Model file for the job. Use its own axes, mm. Round coordinates to 2 decimals unless told otherwise and drop trailing zeros. Write each loop counter-clockwise with the first axis right and the second up, starting at its lowest first coordinate (ties: lowest second). Pieces come first, ordered by that corner, then holes. Notation, with made-up numbers: (-10, 43.5) - (31, 43.5) arc R21 cw to (31, 48.5) - close; hole circle Ø4 at (72, 80). An arc over 180 degrees is marked (long way). One line per item, written item: value.
Autodesk Inventor part; units mm, degrees
ref_plane "YZ Plane" through (0, 0, 0) normal (1, 0, 0) x (0, 1, 0)
ref_plane "XZ Plane" through (0, 0, 0) normal (0, 1, 0) x (-1, 0, 0)
ref_plane "XY Plane" through (0, 0, 0) normal (0, 0, 1) x (1, 0, 0)
sketch "Эскиз1" plane through (0, 0, 0) normal (0, 1, 0) x (-1, 0, 0)
  line L0 (0, 0) -> (30, 0)
  line L1 (30, 0) -> (30, -50)
  line L2 (30, -50) -> (0, -50)
  line L3 (0, -50) -> (0, 0)
  dimension "d0" = 30
  dimension "d1" = 50
extrude "Выдавливание1" add sketch "Эскиз1" along normal blind 15
fillet "Сопряжение1" radius 2 1 edges at (-15, 0, 0)
sketch "Эскиз2" plane through (0, 15, 0) normal (0, 1, 0) x (1, 0, 0)
  line L0 (-30, 0) -> (0, 0)
  point P0 (-15, 20)
  point P1 (-15, 0)
  dimension "d5" = 20
hole "Отверстие1" at (-15, 15, -20) direction (0, -1, 0) diameter 8 end through all
sketch "Эскиз3" plane through (0, 15, 0) normal (0, 1, 0) x (1, 0, 0)
  line L0 (-30, 0) -> (0, 0)
  circle A0 centre (-15, 20) radius 4
  line L1 (-30, 0) -> (0, 0)
  line L2 (0, 0) -> (0, 50)
  line L3 (0, 50) -> (-30, 50)
  line L4 (-30, 50) -> (-30, 0)
  line L5 (-30, 50) -> (-30, 0)
  line L6 (0, 0) -> (0, 50)
  point P0 (-30, 40)
  point P1 (0, 40)
  dimension "d13" = 40
hole "Отверстие2" at (-30, 15, -40) at (0, 15, -40) direction (0, -1, 0) diameter 2 end through all
sketch "Эскиз4" plane through (0, 2, 0) normal (1, 0, 0) x (0, 0, -1)
  line L0 (41, 13) -> (41, -2)
  line L1 (39, 13) -> (41, 13)
  line L2 (39, -2) -> (39, 13)
  line L3 (41, -2) -> (39, -2)
  line L4 (39, 13) -> (41, 13)
  point P0 (0, -2)
  point P1 (40, 13)
hole "Отверстие3" at (0, 15, -40) direction (-1, 0, 0) diameter 2 end through all
properties part number "peg_half" material "Клен"
1. Band-saw the part on D-D on z = -40. Write the cut outline in (x, y).
Report:
outline: (-29, 0) - (-1, 0) - (-1, 14) - (-29, 14) - close
2. Mould opens along Z. For faces 1 (the face through (-30, 7, -19)), 2 (the face through (-18.966, 7.395, -20.521)), 3 (the face through (-15, 8, 0)) say: released by +Z, released by -Z, zero draft, split by the parting line, or undercut.
Report:
face 1: zero draft
face 2: undercut
face 3: released by +Z
3. Band-saw the part on B-B on y = 5.5. Write the cut outline in (x, z).
Report:
outline: (-30, -50) - (0, -50) - (0, -41) arc R1 cw to (0, -39) - (0, 0) - (-30, 0) - (-30, -39) arc R1 cw to (-30, -41) - close; hole circle Ø8 at (-15, -20)
4. Wall check: probe 1 along X at (y, z) = (8, -20); probe 2 along Z at (x, y) = (-14.75, 4.75); probe 3 along Z at (x, y) = (-2.25, 14.5). Give the ranges that are in metal, low to high. Write a range as [from, to].
Report:
probe 1: [-30, -19], [-11, 0]
probe 2: [-50, -23.99], [-16.01, 0]
probe 3: [-50, -40.87], [-39.13, 0]
5. Band-saw the part on C-C on x = -14. Write the cut outline in (y, z).
Report:
outline: (0, -50) - (15, -50) - (15, -41) arc R1 cw to (15, -39) - (15, -23.87) - (0, -23.87) - close; (0, -16.13) - (15, -16.13) - (15, 0) - (2, 0) arc R2 ccw to (0, -2) - close
6. Drop a flat-ended pin along its axis: pin 1 (1.5 mm diameter, centred on x = -14.5, y = 13, fed in from +Z). Give the stop position or say it passes through.
Report:
pin 1: z = 0
7. Band-saw the part on A-A on z = -20. Write the cut outline in (x, y).
Report:
outline: (-30, 0) - (-19, 0) - (-19, 15) - (-30, 15) - close; (-11, 0) - (0, 0) - (0, 15) - (-11, 15) - close
